The figure shows three views and two pictorial views of one solid part (mm, origin at its lowest corner). Answer the questions. A direction names the side the tool comes from. Coordinates: 2 decimals unless noted, no trailing zeros. Order: outer loops, then holes, each group sorted by start corner. A loop starts at its lowest first (then second) coordinate and runs counter-clockwise, first axis right, second up. Notation, with made-up numbers: (-24, -40) - (7, -40) arc R22 ccw to (7, -31) - close; hole circle Ø6 at (66.25, -23). An arc over 180 degrees is marked (long way). Use one line per item in the form item = value. Start each with the question number.
Item 1: Consider line 1 along Z through (x, y) = (15, 1.2); line 2 along X through (y, z) = (12.75, 1.5); line 3 along Z through (x, y) = (27.5, 15.25). Determine where each line is inside the solid, lowest interval first. Write a range as [from, to].
Item 2: The mould has two halves that part along Y. Classify the marked faces 3, 4 and 5: released by +Y, released by -Y, zero draft, split by the parting line, or undercut.
Item 3: Section A-A, the plane y = 10 is taken. Write down the section's boundary in (x, z), and give its area (3 significant figures).
Item 4: Each of these flat-tipped pins is pushed along its axis until it touches: pin 1 Ø5.5 at (x, y) = (21, 12.5) entering from +Z; pin 2 Ø8 at (y, z) = (14, 14) entering from +X; pin 3 Ø5 at (x, z) = (15, 10) entering from +Y; pin 4 Ø9 at (x, z) = (15.5, 12.5) entering from +Y. Where does it stop, or does it pass through?
Item 5: Section B-B, the plane y = 14 is taken. Write down the section's boundary in (x, z), and give its area (3 significant figures).
Item 6: Section D-D, the plane z = 10 is taken. Write down the section's boundary in (x, y), and give its area (3 significant figures).
Item 7: A tool of negligible diameter and unlimited length cuts with its end or side. For the marked faces 1 and 2, from which of +Z, -Z, +X, -X, +Y, -Y can it reach the whole face along a straight path? Write none if from no direction.
Item 8: Section C-C, the plane x = 15 is taken. Write down the section's boundary in (y, z).
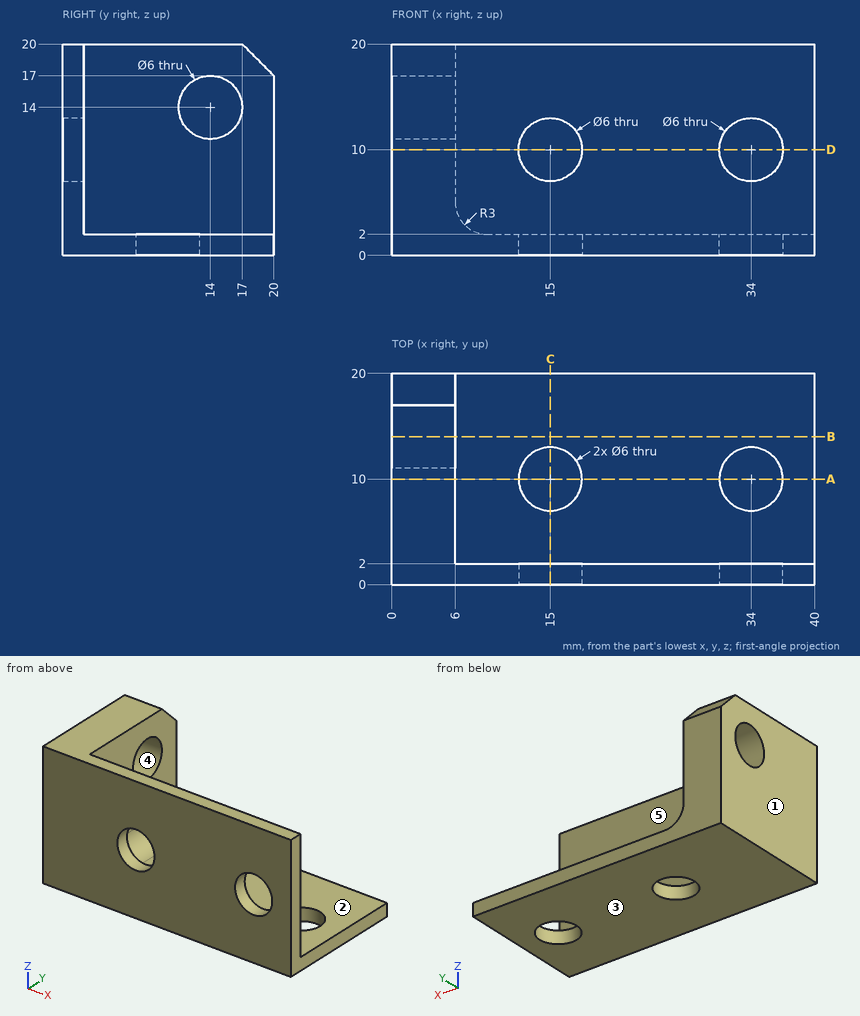
Response:
q1.line_1 = [0, 7], [13, 20]
q1.line_2 = [0, 13.8], [16.2, 32.8], [35.2, 40]
q1.line_3 = [0, 2]
q2.face_3 = zero draft
q2.face_4 = undercut
q2.face_5 = released by +Y
q3.outline = (0, 0) - (12, 0) - (12, 2) - (9, 2) arc R3 cw to (6, 5) - (6, 20) - (0, 20) - close; (18, 0) - (31, 0) - (31, 2) - (18, 2) - close; (37, 0) - (40, 0) - (40, 2) - (37, 2) - close
q3.area = 166 mm2
q4.pin_1 = 2
q4.pin_2 = 6
q4.pin_3 = through
q4.pin_4 = 2
q5.outline = (0, 0) - (40, 0) - (40, 2) - (9, 2) arc R3 cw to (6, 5) - (6, 11) - (0, 11) - close; (0, 17) - (6, 17) - (6, 20) - (0, 20) - close
q5.area = 154 mm2
q6.outline = (0, 0) - (12, 0) - (12, 2) - (6, 2) - (6, 20) - (0, 20) - close; (18, 0) - (31, 0) - (31, 2) - (18, 2) - close; (37, 0) - (40, 0) - (40, 2) - (37, 2) - close
q6.area = 164 mm2
q7.face_1 = +Z, -Z, -X, +Y, -Y
q7.face_2 = +Z, +X, +Y
q8.outline = (0, 0) - (7, 0) - (7, 2) - (2, 2) - (2, 7) - (0, 7) - close; (0, 13) - (2, 13) - (2, 20) - (0, 20) - close; (13, 0) - (20, 0) - (20, 2) - (13, 2) - close
